Design review of the part built by this model. Coordinates are the model's own, in mm. Face numbers are marked on the shaded views. A direction names the side the tool comes from. Coordinates: 2 decimals unless noted, no trailing zeros. Loops run counter-clockwise (first coordinate to the right, second up) from the corner with the lowest first, then second, coordinate; pieces in that order, holes last. Notation, with made-up numbers: (18.5, 37) -> (58.5, 37) arc R10 cw to (58.5, 51) -> close; hole circle Ø7 at (50, 45.25). An arc over 180 degrees is marked (long way). Answer in a Markdown table with one row per item.
```python
from build123d import *

# Parameters (mm, degrees)
SKETCH1_W                = 127.76
SKETCH1_H                = 85.48
BOSS_EXTRUDE1_DEPTH      = 5
SKETCH2_R                = 10.875
CUT_EXTRUDE1_DEPTH       = 95.825210988
SKETCH3_W                = 5
SKETCH3_H                = 5
BOSS_EXTRUDE2_DEPTH      = 25
LPATTERN2_COUNT          = 4
LPATTERN2_PITCH          = 30
LPATTERN2_COUNT_DIR2     = 3
LPATTERN2_PITCH_DIR2     = 27
LPATTERN3_COUNT          = 5
LPATTERN3_PITCH          = 30.65
LPATTERN3_COUNT_DIR2     = 4
LPATTERN3_PITCH_DIR2     = 26.75
MIRROR5_START            = -54.673764706
MIRROR5_OUTLINE_W        = 5
MIRROR5_OUTLINE_H        = 25
MIRROR5_DEPTH            = 5
MIRROR5_START_2          = -24.023764706
MIRROR5_2_OUTLINE_W      = 5
MIRROR5_2_OUTLINE_H      = 25
MIRROR5_2_DEPTH          = 5
MIRROR5_START_3          = 6.626235294
MIRROR5_3_OUTLINE_W      = 5
MIRROR5_3_OUTLINE_H      = 25
MIRROR5_3_DEPTH          = 5
MIRROR5_START_4          = 37.276235294
MIRROR5_4_OUTLINE_W      = 5
MIRROR5_4_OUTLINE_H      = 25
MIRROR5_4_DEPTH          = 5
MIRROR5_START_5          = 67.926235294
MIRROR5_5_OUTLINE_W      = 5
MIRROR5_5_OUTLINE_H      = 25
MIRROR5_5_DEPTH          = 5
MIRROR6_COPY_1_SKETCH_R  = 10.875
MIRROR6_COPY_1_DEPTH     = 95.825210988
MIRROR6_COPY_2_SKETCH_R  = 10.875
MIRROR6_COPY_2_DEPTH     = 95.825210988
MIRROR6_COPY_3_SKETCH_R  = 10.875
MIRROR6_COPY_3_DEPTH     = 95.825210988
MIRROR6_COPY_4_SKETCH_R  = 10.875
MIRROR6_COPY_4_DEPTH     = 95.825210988
MIRROR6_COPY_5_SKETCH_R  = 10.875
MIRROR6_COPY_5_DEPTH     = 95.825210988
MIRROR6_COPY_6_SKETCH_R  = 10.875
MIRROR6_COPY_6_DEPTH     = 95.825210988
MIRROR6_COPY_7_SKETCH_R  = 10.875
MIRROR6_COPY_7_DEPTH     = 95.825210988
MIRROR6_COPY_8_SKETCH_R  = 10.875
MIRROR6_COPY_8_DEPTH     = 95.825210988
MIRROR6_COPY_9_SKETCH_R  = 10.875
MIRROR6_COPY_9_DEPTH     = 95.825210988
MIRROR6_COPY_10_SKETCH_R = 10.875
MIRROR6_COPY_10_DEPTH    = 95.825210988
MIRROR6_COPY_11_SKETCH_R = 10.875
MIRROR6_COPY_11_DEPTH    = 95.825210988


# Read off the part's stored shape, not the designer's step: Mirror5
with BuildPart() as part:
    # Sketch1 → Boss-Extrude1 (new body)
    with BuildSketch(Plane.XY):
        with Locations((9.206235294, -17.469823529)):
            Rectangle(SKETCH1_W, SKETCH1_H)
    boss_extrude1 = extrude(amount=BOSS_EXTRUDE1_DEPTH)

    # Sketch2 → Cut-Extrude1 (cut, through all)
    with BuildSketch(Plane.XY.offset(5)):
        with Locations((-35.793764706, 9.530176471)):
            Circle(SKETCH2_R)
    cut_extrude1 = extrude(amount=-CUT_EXTRUDE1_DEPTH, mode=Mode.SUBTRACT)

    # Sketch3 → Boss-Extrude2 (add)
    with BuildSketch(Plane.XY.offset(5)):
        with Locations((-52.173764706, 22.770176471)):
            Rectangle(SKETCH3_W, SKETCH3_H)
    boss_extrude2 = extrude(amount=BOSS_EXTRUDE2_DEPTH)

    # LPattern2: Cut-Extrude1 4 × 3
    with Locations(*[(i * LPATTERN2_PITCH, -j * LPATTERN2_PITCH_DIR2, 0) for i in range(LPATTERN2_COUNT) for j in range(LPATTERN2_COUNT_DIR2) if (i, j) != (0, 0)]):
        add(cut_extrude1, mode=Mode.SUBTRACT)

    # LPattern3: Boss-Extrude2 5 × 4
    with Locations(*[(i * LPATTERN3_PITCH, -j * LPATTERN3_PITCH_DIR2, 0) for i in range(LPATTERN3_COUNT) for j in range(LPATTERN3_COUNT_DIR2) if (i, j) != (0, 0)]):
        add(boss_extrude2)

    # Mirror5 outline → Mirror5 (add)
    with BuildSketch(Plane.YZ.offset(MIRROR5_START)):
        with Locations((22.770176471, 42.5)):
            Rectangle(MIRROR5_OUTLINE_W, MIRROR5_OUTLINE_H)
        with Locations((-3.979823529, 42.5)):
            Rectangle(MIRROR5_OUTLINE_W, MIRROR5_OUTLINE_H)
        with Locations((-30.729823529, 42.5)):
            Rectangle(MIRROR5_OUTLINE_W, MIRROR5_OUTLINE_H)
        with Locations((-57.479823529, 42.5)):
            Rectangle(MIRROR5_OUTLINE_W, MIRROR5_OUTLINE_H)
    extrude(amount=MIRROR5_DEPTH)

    # Mirror5 2 outline → Mirror5 2 (add)
    with BuildSketch(Plane.YZ.offset(MIRROR5_START_2)):
        with Locations((22.770176471, 42.5)):
            Rectangle(MIRROR5_2_OUTLINE_W, MIRROR5_2_OUTLINE_H)
        with Locations((-3.979823529, 42.5)):
            Rectangle(MIRROR5_2_OUTLINE_W, MIRROR5_2_OUTLINE_H)
        with Locations((-30.729823529, 42.5)):
            Rectangle(MIRROR5_2_OUTLINE_W, MIRROR5_2_OUTLINE_H)
        with Locations((-57.479823529, 42.5)):
            Rectangle(MIRROR5_2_OUTLINE_W, MIRROR5_2_OUTLINE_H)
    extrude(amount=MIRROR5_2_DEPTH)

    # Mirror5 3 outline → Mirror5 3 (add)
    with BuildSketch(Plane.YZ.offset(MIRROR5_START_3)):
        with Locations((22.770176471, 42.5)):
            Rectangle(MIRROR5_3_OUTLINE_W, MIRROR5_3_OUTLINE_H)
        with Locations((-3.979823529, 42.5)):
            Rectangle(MIRROR5_3_OUTLINE_W, MIRROR5_3_OUTLINE_H)
        with Locations((-30.729823529, 42.5)):
            Rectangle(MIRROR5_3_OUTLINE_W, MIRROR5_3_OUTLINE_H)
        with Locations((-57.479823529, 42.5)):
            Rectangle(MIRROR5_3_OUTLINE_W, MIRROR5_3_OUTLINE_H)
    extrude(amount=MIRROR5_3_DEPTH)

    # Mirror5 4 outline → Mirror5 4 (add)
    with BuildSketch(Plane.YZ.offset(MIRROR5_START_4)):
        with Locations((22.770176471, 42.5)):
            Rectangle(MIRROR5_4_OUTLINE_W, MIRROR5_4_OUTLINE_H)
        with Locations((-3.979823529, 42.5)):
            Rectangle(MIRROR5_4_OUTLINE_W, MIRROR5_4_OUTLINE_H)
        with Locations((-30.729823529, 42.5)):
            Rectangle(MIRROR5_4_OUTLINE_W, MIRROR5_4_OUTLINE_H)
        with Locations((-57.479823529, 42.5)):
            Rectangle(MIRROR5_4_OUTLINE_W, MIRROR5_4_OUTLINE_H)
    extrude(amount=MIRROR5_4_DEPTH)

    # Mirror5 5 outline → Mirror5 5 (add)
    with BuildSketch(Plane.YZ.offset(MIRROR5_START_5)):
        with Locations((22.770176471, 42.5)):
            Rectangle(MIRROR5_5_OUTLINE_W, MIRROR5_5_OUTLINE_H)
        with Locations((-3.979823529, 42.5)):
            Rectangle(MIRROR5_5_OUTLINE_W, MIRROR5_5_OUTLINE_H)
        with Locations((-30.729823529, 42.5)):
            Rectangle(MIRROR5_5_OUTLINE_W, MIRROR5_5_OUTLINE_H)
        with Locations((-57.479823529, 42.5)):
            Rectangle(MIRROR5_5_OUTLINE_W, MIRROR5_5_OUTLINE_H)
    extrude(amount=MIRROR5_5_DEPTH)

    # Mirror6: Boss-Extrude1, Cut-Extrude1 across plane
    add(boss_extrude1.mirror(Plane(origin=(0, 0, 30), x_dir=(1, 0, 0), z_dir=(0, 0, -1))))
    add(cut_extrude1.mirror(Plane(origin=(0, 0, 30), x_dir=(1, 0, 0), z_dir=(0, 0, -1))), mode=Mode.SUBTRACT)

    # Mirror6 copy 1 sketch → Mirror6 copy 1 (cut, through all)
    with BuildSketch(Plane(origin=(0, -27, 55), x_dir=(1, 0, 0), z_dir=(0, 0, -1))):
        with Locations((-35.793764706, -9.530176471)):
            Circle(MIRROR6_COPY_1_SKETCH_R)
    extrude(amount=-MIRROR6_COPY_1_DEPTH, mode=Mode.SUBTRACT)

    # Mirror6 copy 2 sketch → Mirror6 copy 2 (cut, through all)
    with BuildSketch(Plane(origin=(0, -54, 55), x_dir=(1, 0, 0), z_dir=(0, 0, -1))):
        with Locations((-35.793764706, -9.530176471)):
            Circle(MIRROR6_COPY_2_SKETCH_R)
    extrude(amount=-MIRROR6_COPY_2_DEPTH, mode=Mode.SUBTRACT)

    # Mirror6 copy 3 sketch → Mirror6 copy 3 (cut, through all)
    with BuildSketch(Plane(origin=(30, 0, 55), x_dir=(1, 0, 0), z_dir=(0, 0, -1))):
        with Locations((-35.793764706, -9.530176471)):
            Circle(MIRROR6_COPY_3_SKETCH_R)
    extrude(amount=-MIRROR6_COPY_3_DEPTH, mode=Mode.SUBTRACT)

    # Mirror6 copy 4 sketch → Mirror6 copy 4 (cut, through all)
    with BuildSketch(Plane(origin=(30, -27, 55), x_dir=(1, 0, 0), z_dir=(0, 0, -1))):
        with Locations((-35.793764706, -9.530176471)):
            Circle(MIRROR6_COPY_4_SKETCH_R)
    extrude(amount=-MIRROR6_COPY_4_DEPTH, mode=Mode.SUBTRACT)

    # Mirror6 copy 5 sketch → Mirror6 copy 5 (cut, through all)
    with BuildSketch(Plane(origin=(30, -54, 55), x_dir=(1, 0, 0), z_dir=(0, 0, -1))):
        with Locations((-35.793764706, -9.530176471)):
            Circle(MIRROR6_COPY_5_SKETCH_R)
    extrude(amount=-MIRROR6_COPY_5_DEPTH, mode=Mode.SUBTRACT)

    # Mirror6 copy 6 sketch → Mirror6 copy 6 (cut, through all)
    with BuildSketch(Plane(origin=(60, 0, 55), x_dir=(1, 0, 0), z_dir=(0, 0, -1))):
        with Locations((-35.793764706, -9.530176471)):
            Circle(MIRROR6_COPY_6_SKETCH_R)
    extrude(amount=-MIRROR6_COPY_6_DEPTH, mode=Mode.SUBTRACT)

    # Mirror6 copy 7 sketch → Mirror6 copy 7 (cut, through all)
    with BuildSketch(Plane(origin=(60, -27, 55), x_dir=(1, 0, 0), z_dir=(0, 0, -1))):
        with Locations((-35.793764706, -9.530176471)):
            Circle(MIRROR6_COPY_7_SKETCH_R)
    extrude(amount=-MIRROR6_COPY_7_DEPTH, mode=Mode.SUBTRACT)

    # Mirror6 copy 8 sketch → Mirror6 copy 8 (cut, through all)
    with BuildSketch(Plane(origin=(60, -54, 55), x_dir=(1, 0, 0), z_dir=(0, 0, -1))):
        with Locations((-35.793764706, -9.530176471)):
            Circle(MIRROR6_COPY_8_SKETCH_R)
    extrude(amount=-MIRROR6_COPY_8_DEPTH, mode=Mode.SUBTRACT)

    # Mirror6 copy 9 sketch → Mirror6 copy 9 (cut, through all)
    with BuildSketch(Plane(origin=(90, 0, 55), x_dir=(1, 0, 0), z_dir=(0, 0, -1))):
        with Locations((-35.793764706, -9.530176471)):
            Circle(MIRROR6_COPY_9_SKETCH_R)
    extrude(amount=-MIRROR6_COPY_9_DEPTH, mode=Mode.SUBTRACT)

    # Mirror6 copy 10 sketch → Mirror6 copy 10 (cut, through all)
    with BuildSketch(Plane(origin=(90, -27, 55), x_dir=(1, 0, 0), z_dir=(0, 0, -1))):
        with Locations((-35.793764706, -9.530176471)):
            Circle(MIRROR6_COPY_10_SKETCH_R)
    extrude(amount=-MIRROR6_COPY_10_DEPTH, mode=Mode.SUBTRACT)

    # Mirror6 copy 11 sketch → Mirror6 copy 11 (cut, through all)
    with BuildSketch(Plane(origin=(90, -54, 55), x_dir=(1, 0, 0), z_dir=(0, 0, -1))):
        with Locations((-35.793764706, -9.530176471)):
            Circle(MIRROR6_COPY_11_SKETCH_R)
    extrude(amount=-MIRROR6_COPY_11_DEPTH, mode=Mode.SUBTRACT)


solid = part.part
```
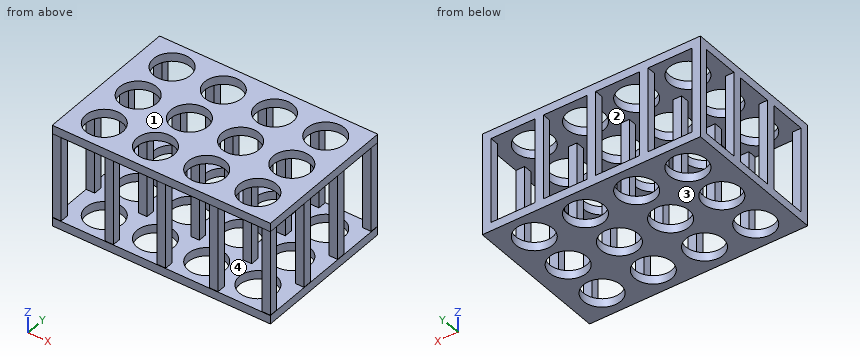
(1) To check wall thickness, follow probe 1 along Y at (x, z) = (7, 49.5); probe 2 along X at (y, z) = (21, 17); probe 3 along Z at (x, y) = (60, -2.5). State the ranges of each line that lie inside material, in increasing order.
Evaluation:
| item | result |
|---|---|
| probe 1 | y = -59.98 to -54.98, -33.23 to -28.23, -6.48 to -1.48, 20.27 to 25.27 |
| probe 2 | x = -54.67 to -49.67, -24.02 to -19.02, 6.63 to 11.63, 37.28 to 42.28, 67.93 to 72.93 |
| probe 3 | z = 0 to 5, 55 to 60 |
(2) Take a section at A-A on x = -21. Give the boundary of the cut face in (y, z).
Evaluation:
| item | result |
|---|---|
| outline | (-60.21, 0) -> (25.27, 0) -> (25.27, 60) -> (-60.21, 60) -> (-60.21, 55) -> (-59.98, 55) -> (-59.98, 5) -> (-60.21, 5) -> close; hole (-54.98, 5) -> (-33.23, 5) -> (-33.23, 55) -> (-54.98, 55) -> close; hole (-28.23, 5) -> (-6.48, 5) -> (-6.48, 55) -> (-28.23, 55) -> close; hole (-1.48, 5) -> (20.27, 5) -> (20.27, 55) -> (-1.48, 55) -> close |
(3) Take a section at B-B on z = 37. Count the separate pieces of the cut face and the enclosed holes in it, and give its area (3 significant figures).
Evaluation:
| item | result |
|---|---|
| separate pieces | 20 |
| enclosed holes | 0 |
| area | 500 mm² |
(4) For pin 1 (5.5 mm diameter, centred on x = -21.5, z = 34, fed in from -Y); pin 2 (4 mm diameter, centred on y = 23.5, z = 21.5, fed in from +X); pin 3 (5 mm diameter, centred on y = -28, z = 49, fed in from -X); pin 4 (5 mm diameter, centred on x = 26, y = 2, fed in from -Z), all flat-tipped, find the tip position at first contact; note any pin that passes through.
Evaluation:
| item | result |
|---|---|
| pin 1 | stops at y = -59.98 |
| pin 2 | stops at x = 72.93 |
| pin 3 | stops at x = -54.67 |
| pin 4 | passes through |
(5) Tool access review of the marked faces 1 and 2: name each direction out of +Z, -Z, +X, -X, +Y, -Y from which nothing blocks a thin tool from reaching the whole face with its end or side.
Evaluation:
| item | result |
|---|---|
| face 1 | +Z, +X, -X, +Y, -Y |
| face 2 | none |
(6) Draft analysis for pull direction Y (two halves, no side actions). For the marked faces 3 and 4, state which applies: pulls with the +Y half, pulls with the -Y half, needs draft (parallel to the pull), parting line crosses it, or undercut.
Evaluation:
| item | result |
|---|---|
| face 3 | needs draft |
| face 4 | undercut |
